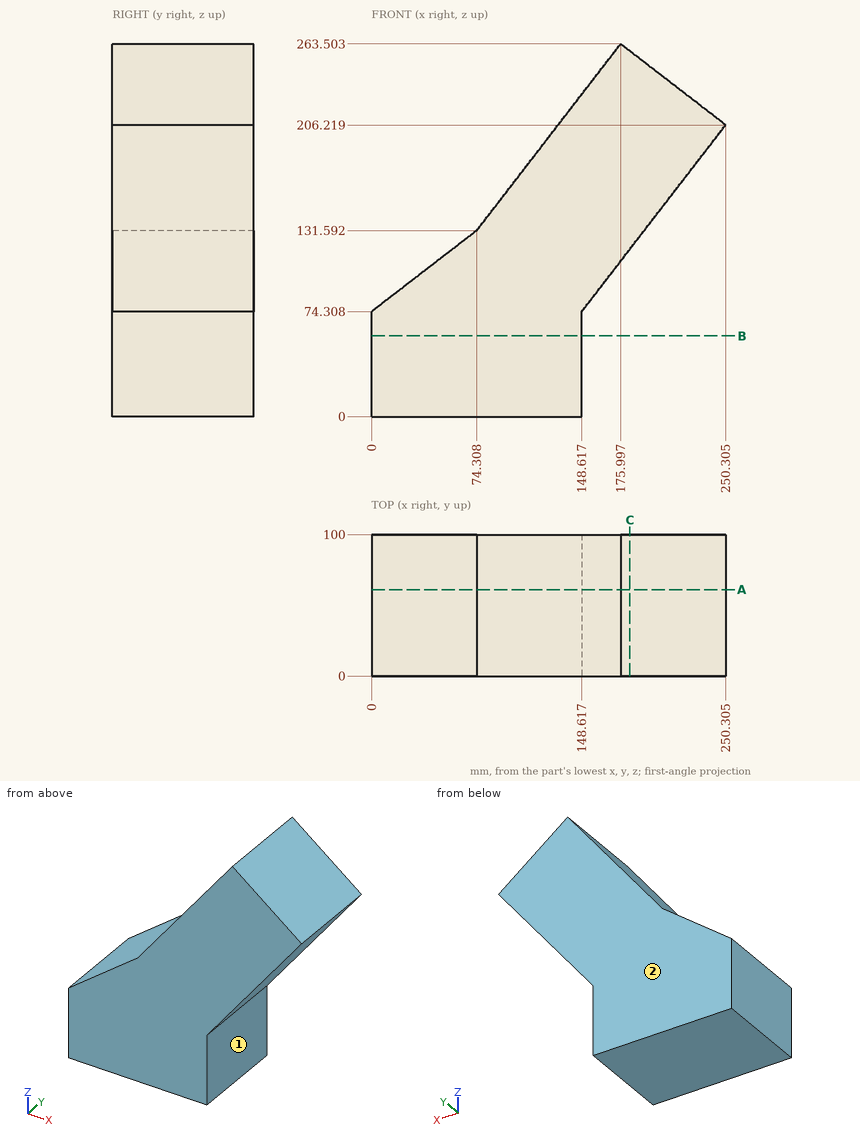
Job drawing, mm, ordinate dimensions from the low corner. One solid piece. A direction names the side the tool comes from. Give positions to 0.01 mm unless a question says otherwise; leave off trailing zeros. Order: outer loops, then holes, each group sorted by start corner. A loop starts at its lowest first (then second) coordinate and runs counter-clockwise, first axis right, second up. Notation, with made-up numbers: (27, 67) -> (59, 67) arc R28 ccw to (59, 101) -> close; hole circle Ø2 at (-37.75, 20). An arc over 180 degrees is marked (long way). Return JSON: item names as keys, results as strings.
Q1. Flat gauge pins, fed straight in: pin 1 (1 mm diameter, centred on y = 23, z = 222, fed in from -X); pin 2 (8 mm diameter, centred on x = 83.5, y = 51, fed in from -Z); pin 3 (5 mm diameter, centred on x = 223, y = 70, fed in from -Z) (1 decimal); pin 4 (1 mm diameter, centred on y = 75.5, z = 166, fed in from -X). Where does each tip first touch, or does it go through?
Working result:
{"pin 1": "x = 143.62", "pin 2": "z = 0", "pin 3": "z = 167.6", "pin 4": "x = 100.45"}
Q2. Drill centre lines: line 1 (X direction, y = 29, z = 50); line 2 (Z direction, x = 226.5, y = 78); line 3 (Z direction, x = 91, y = 68) (1 decimal). Where is each one in solid material? Low to high.
Working result:
{"line 1": "0 to 148.62", "line 2": "175.34 to 224.57", "line 3": "0 to 153.2"}
Q3. Saw through at B-B (z = 57). Write the cut outline in (x, y).
Working result:
{"outline": "(0, 0) -> (148.62, 0) -> (148.62, 100) -> (0, 100) -> close"}
Q4. Saw through at C-C (x = 182.5). Write the cut outline in (y, z), then the cut area to 3 significant figures.
Working result:
{"outline": "(0, 118.26) -> (100, 118.26) -> (100, 258.49) -> (0, 258.49) -> close", "area": "14,000 mm²"}
Q5. Which spindle directions (+Z, -Z, +X, -X, +Y, -Y) get a long thin tool onto all of the face, cutting with end or side? Do the marked faces 1 and 2. Say none if no direction does.
Working result:
{"face 1": "-Z, +X, +Y, -Y", "face 2": "+Z, -Z, +X, -X, +Y"}
Q6. Saw through at A-A (y = 61). Write the cut outline in (x, z) (1 decimal), then the cut area to 3 significant figures.
Working result:
{"outline": "(0, 0) -> (148.6, 0) -> (148.6, 74.3) -> (250.3, 206.2) -> (176, 263.5) -> (74.3, 131.6) -> (0, 74.3) -> close", "area": "30,900 mm²"}
